```python
from build123d import *

# Parameters (mm, degrees)
SKETCH1_W            = 1250
SKETCH1_H            = 2500
BOSS_EXTRUDE1_DEPTH  = 200
SKETCH2_W            = 1240
SKETCH2_H            = 2490
CUT_EXTRUDE1_DEPTH   = 190
BOSS_EXTRUDE2_DEPTH  = 200
SKETCH8_W            = 10
SKETCH8_H            = 250
BOSS_EXTRUDE3_DEPTH  = 200
SKETCH10_W           = 250
SKETCH10_H           = 10
BOSS_EXTRUDE4_DEPTH  = 200
BOSS_EXTRUDE8_DEPTH  = 200
SKETCH11_W           = 250
SKETCH11_H           = 10
BOSS_EXTRUDE5_DEPTH  = 200
SKETCH12_W           = 250
SKETCH12_H           = 10
BOSS_EXTRUDE6_DEPTH  = 200
SKETCH18_W           = 250
SKETCH18_H           = 10
BOSS_EXTRUDE9_DEPTH  = 10
BOSS_EXTRUDE10_DEPTH = 200
SKETCH23_W           = 50
SKETCH23_H           = 250
BOSS_EXTRUDE11_DEPTH = 200
SKETCH24_W           = 250
SKETCH24_H           = 50
BOSS_EXTRUDE12_DEPTH = 200
SKETCH25_W           = 250
SKETCH25_H           = 50
BOSS_EXTRUDE13_DEPTH = 200
SKETCH26_W           = 55
SKETCH26_H           = 250
BOSS_EXTRUDE14_DEPTH = 200


with BuildPart() as part:
    # Sketch1 → Boss-Extrude1 (new body)
    with BuildSketch(Plane(origin=(0, 0, 0), x_dir=(1, 0, 0), z_dir=(0, 1, 0))):
        Rectangle(SKETCH1_W, SKETCH1_H)
    extrude(amount=BOSS_EXTRUDE1_DEPTH)

    # Sketch2 → Cut-Extrude1 (cut)
    with BuildSketch(Plane(origin=(0, 200, 0), x_dir=(1, 0, 0), z_dir=(0, 1, 0))):
        Rectangle(SKETCH2_W, SKETCH2_H)
    extrude(amount=-CUT_EXTRUDE1_DEPTH, mode=Mode.SUBTRACT)

    # Sketch7 → Boss-Extrude2 (add)
    with BuildSketch(Plane(origin=(0, 10, 0), x_dir=(1, 0, 0), z_dir=(0, 1, 0))):
        Polygon((-170, -705), (-270, -705), (-270, -715), (-117.906694844, -715), (-70, -715), (-70, -705), align=None)
    extrude(amount=BOSS_EXTRUDE2_DEPTH)

    # Sketch8 → Boss-Extrude3 (add)
    with BuildSketch(Plane(origin=(0, 10, 0), x_dir=(1, 0, 0), z_dir=(0, 1, 0))):
        with Locations((-170, -840)):
            Rectangle(SKETCH8_W, SKETCH8_H)
    extrude(amount=BOSS_EXTRUDE3_DEPTH)

    # Sketch10 → Boss-Extrude4 (add)
    with BuildSketch(Plane(origin=(0, 10, 0), x_dir=(1, 0, 0), z_dir=(0, 1, 0))):
        with Locations((-495, -5)):
            Rectangle(SKETCH10_W, SKETCH10_H)
    extrude(amount=BOSS_EXTRUDE4_DEPTH)

    # Sketch17 → Boss-Extrude8 (add)
    with BuildSketch(Plane(origin=(0, 10, 0), x_dir=(1, 0, 0), z_dir=(0, 1, 0))):
        Polygon((0, 200), (-75, 0), (0, -200), (75, 0), align=None)
    extrude(amount=BOSS_EXTRUDE8_DEPTH)

    # Sketch11 → Boss-Extrude5 (add)
    with BuildSketch(Plane(origin=(0, 10, 0), x_dir=(1, 0, 0), z_dir=(0, 1, 0))):
        with Locations((495, -5)):
            Rectangle(SKETCH11_W, SKETCH11_H)
    extrude(amount=BOSS_EXTRUDE5_DEPTH)

    # Sketch12 → Boss-Extrude6 (add)
    with BuildSketch(Plane(origin=(0, 10, 0), x_dir=(1, 0, 0), z_dir=(0, 1, 0))):
        with Locations((495, -415)):
            Rectangle(SKETCH12_W, SKETCH12_H)
    extrude(amount=BOSS_EXTRUDE6_DEPTH)

    # Sketch18 → Boss-Extrude9 (add)
    with BuildSketch(Plane(origin=(0, 10, 0), x_dir=(1, 0, 0), z_dir=(0, 1, 0))):
        with Locations((-495, 405)):
            Rectangle(SKETCH18_W, SKETCH18_H)
    extrude(amount=BOSS_EXTRUDE9_DEPTH)

    # Sketch21 → Boss-Extrude10 (add)
    with BuildSketch(Plane(origin=(0, 10, 0), x_dir=(1, 0, 0), z_dir=(0, 1, 0))):
        Polygon((170, 710), (328.507885592, 710), (328.507885592, 720), (233.507885592, 720), (233.507885592, 960), (223.507885592, 960), (223.507885592, 720), (128.507885592, 720), (128.507885592, 710), align=None)
    extrude(amount=BOSS_EXTRUDE10_DEPTH)

    # Sketch23 → Boss-Extrude11 (add)
    with BuildSketch(Plane(origin=(0, 10, 0), x_dir=(1, 0, 0), z_dir=(0, 1, 0))):
        with Locations((-595, -1120)):
            Rectangle(SKETCH23_W, SKETCH23_H)
    extrude(amount=BOSS_EXTRUDE11_DEPTH)

    # Sketch24 → Boss-Extrude12 (add)
    with BuildSketch(Plane(origin=(0, 10, 0), x_dir=(1, 0, 0), z_dir=(0, 1, 0))):
        with Locations((5, -1220)):
            Rectangle(SKETCH24_W, SKETCH24_H)
    extrude(amount=BOSS_EXTRUDE12_DEPTH)

    # Sketch25 → Boss-Extrude13 (add)
    with BuildSketch(Plane(origin=(0, 10, 0), x_dir=(1, 0, 0), z_dir=(0, 1, 0))):
        with Locations((-495, 1220)):
            Rectangle(SKETCH25_W, SKETCH25_H)
    extrude(amount=BOSS_EXTRUDE13_DEPTH)

    # Sketch26 → Boss-Extrude14 (add)
    with BuildSketch(Plane(origin=(0, 10, 0), x_dir=(1, 0, 0), z_dir=(0, 1, 0))):
        with Locations((597.5, 269.101726834)):
            Rectangle(SKETCH26_W, SKETCH26_H)
    extrude(amount=BOSS_EXTRUDE14_DEPTH)


solid = part.part
```
The model under review builds one solid part; all positions refer to its coordinate system, in mm. A direction names the side the tool comes from. Give positions to 0.01 mm unless a question says otherwise; leave off trailing zeros. Order: outer loops, then holes, each group sorted by start corner. A loop starts at its lowest first (then second) coordinate and runs counter-clockwise, first axis right, second up. Notation, with made-up numbers: (68, 17.25) - (106, 17.25) arc R9 ccw to (106, 28.25) - close; hole circle Ø6 at (-10.75, 34). An arc over 180 degrees is marked (long way). Use CSV: the item, a comma, the result in double quotes. Start each with the question number.
Q1. To check wall thickness, follow line 1 along X through (y, z) = (155.5, 922); line 2 along Z through (x, y) = (132, 101); line 3 along Z through (x, y) = (407, 46). State the ranges of each line that lie inside material, in increasing order. Write a range as [from, to].
Q2. We need section A-A, the plane y = 159. State how many separate pieces and enclosed holes the cut face has, and give its area (3 significant figures).
Q3. The part is to be moulded in two halves that separate along X. For faces 3 (the flat face through (625, 104, 17)), 4 (the flat face through (-9, 0, -18)), 5 (the flat face through (-620, 106, 509)), say which applies: +X half, -X half, draft (parallel to the pull), parting line (faces both ways), or undercut.
Q4. Tool access review of faces 1 (the flat face through (-497, 210, -1220)), 2 (the flat face through (-38.025, 108.6, 98.6)): name each direction out of +Z, -Z, +X, -X, +Y, -Y from which nothing blocks a thin tool from reaching the whole face with its end or side.
Q5. We need section B-B, the plane x = -313. Write out the cut boundary in (y, z), and give its area (3 significant figures).
Q6. We need section D-D, the plane z = 918.5. Write out the cut boundary in (x, y), and give its area (3 significant figures).
Q7. Clearance check with flat-ended pins moving along their axes: pin 1 Ø2 at (x, z) = (-343, 735.5) entering from +Y; pin 2 Ø11 at (x, z) = (-462.5, -407) entering from +Y; pin 3 Ø8 at (y, z) = (202.5, 7) entering from -X. State where each tip first meets the part, or that it passes through.
Q8. We need section C-C, the plane z = -1019. Write out the cut boundary in (x, y).
Outcome:
1,line 1,"x = [-625, -620], [-175, -165], [620, 625]"
1,line 2,"z = [-1250, -1245], [-720, -710], [1245, 1250]"
1,line 3,"z = [-1250, -1245], [0, 10], [410, 420], [1245, 1250]"
2,separate pieces,"4"
2,enclosed holes,"1"
2,area,"134,000 mm^2"
3,face 3,"+X half"
3,face 4,"draft"
3,face 5,"undercut"
4,face 1,"+Z, -Z, +X, -X, +Y"
4,face 2,"+Y"
5,outline,"(0, -1250) - (200, -1250) - (200, -1245) - (10, -1245) - (10, 1245) - (200, 1245) - (200, 1250) - (0, 1250) - close"
5,area,"26,900 mm^2"
6,outline,"(-625, 0) - (625, 0) - (625, 200) - (620, 200) - (620, 10) - (-165, 10) - (-165, 210) - (-175, 210) - (-175, 10) - (-620, 10) - (-620, 200) - (-625, 200) - close"
6,area,"16,400 mm^2"
7,pin 1,"stops at y = 10"
7,pin 2,"stops at y = 20"
7,pin 3,"stops at x = -625"
8,outline,"(-625, 0) - (625, 0) - (625, 200) - (620, 200) - (620, 10) - (-620, 10) - (-620, 200) - (-625, 200) - close"
